Can you work these out from the model? Positions are in its coordinate system, mm. A direction names the side the tool comes from. Coordinates: 2 decimals unless noted, no trailing zeros. Loops run counter-clockwise (first coordinate to the right, second up) from the corner with the lowest first, then second, coordinate; pieces in that order, holes last. Notation, with made-up numbers: M 65.5,36 L 96.5,36 A26 ccw 96.5,53 Z; hole C -19.75,32 d5. An arc over 180 degrees is marked long. Answer as a JSON object with one key per item and string values. Group by question number.
Item 1: If I drill on line 1 (Z direction, x = 25.4, y = 3.25); line 2 (X direction, y = 8.5, z = -73); line 3 (X direction, y = 7, z = -31.75), over which ranges is the centre line in solid material (lowest first)?
Item 2: Which directions (+Z, -Z, +X, -X, +Y, -Y) give clear straight access to the entire face, cutting with the end or side of a thin tool? Please do faces 3 (the flat face through (684, 0, -177)), 4 (the flat face through (295.988, 5.009, -186.063)).
Item 3: We'd pull the mould along X, two halves only. Please class faces 1 (the flat face through (1165.75, 5.01, -178.62)), 2 (the flat face through (684, 10.16, -177)): +X half, -X half, draft (parallel to the pull), parting line (faces both ways), or undercut.
Item 4: I'm going to push a flat-ended pin straight in: pin 1 Ø7.5 at (x, z) = (1361.53, -31.75) entering from +Y. Where does the tip first touch, or does it pass through?
Item 5: Suppose I cut it at A-A (x = 337.5). Write out the boundary of the cut face in (y, z).
Item 6: Suppose I cut it at B-B (y = 2.25). Count the separate pieces of the cut face and the enclosed holes in it, then the cut area to 3 significant figures.
```python
from build123d import *

# Parameters (mm, degrees)
SKETCH1_W           = 1386.9289
SKETCH1_H           = 349.25
SKETCH1_W_2         = 1285.3289
SKETCH1_H_2         = 247.65
BOSS_EXTRUDE1_DEPTH = 10.16
FILLET1_R           = 19.05
SKETCH4_R           = 4.7625
CUT_EXTRUDE1_DEPTH  = 11.16


with BuildPart() as part:
    # Sketch1 → Boss-Extrude1 (new body)
    with BuildSketch(Plane(origin=(0, 0, 0), x_dir=(1, 0, 0), z_dir=(0, 1, 0))):
        with Locations((693.46445, 174.625)):
            Rectangle(SKETCH1_W, SKETCH1_H)
        with Locations((693.46445, 174.625)):
            Rectangle(SKETCH1_W_2, SKETCH1_H_2, mode=Mode.SUBTRACT)
        Polygon((453.842966667, 65.481790785), (50.8, 298.45), (50.8, 269.112055616), (428.487319876, 50.8), (453.842966667, 50.8), align=None)
        Polygon((101.55564679, 298.45), (50.8, 298.45), (453.842966667, 65.481790785), (453.842966667, 94.819735169), align=None)
        Polygon((453.842966667, 94.819735169), (453.842966667, 65.481790785), (453.842966667, 50.8), (479.242966667, 50.8), (479.242966667, 298.45), (453.842966667, 298.45), align=None)
        Polygon((504.642966667, 298.45), (479.242966667, 298.45), (479.242966667, 50.8), (504.642966667, 50.8), (504.642966667, 65.481790785), (504.642966667, 94.819735169), align=None)
        Polygon((882.285933333, 298.45), (856.930286543, 298.45), (504.642966667, 94.819735169), (504.642966667, 65.481790785), (882.285933333, 283.768209215), align=None)
        Polygon((504.642966667, 65.481790785), (504.642966667, 50.8), (529.998613457, 50.8), (882.285933333, 254.430264831), (882.285933333, 283.768209215), align=None)
        Polygon((907.685933333, 298.45), (882.285933333, 298.45), (882.285933333, 283.768209215), (882.285933333, 254.430264831), (882.285933333, 50.8), (907.685933333, 50.8), align=None)
        Polygon((933.085933333, 298.45), (907.685933333, 298.45), (907.685933333, 50.8), (933.085933333, 50.8), (933.085933333, 254.430264831), (933.085933333, 283.768209215), align=None)
        Polygon((1336.1289, 50.8), (933.085933333, 283.768209215), (933.085933333, 254.430264831), (1285.37325321, 50.8), align=None)
        Polygon((958.441580124, 298.45), (933.085933333, 298.45), (933.085933333, 283.768209215), (1336.1289, 50.8), (1336.1289, 80.137944384), align=None)
    extrude(amount=BOSS_EXTRUDE1_DEPTH)

    # Fillet1
    fillet1_edges = [part.edges().sort_by_distance(p)[0] for p in [
        (428.487319876, 5.08, -50.8),
        (50.8, 5.08, -269.112055616),
        (50.8, 5.08, -50.8),
        (1336.1289, 5.08, -80.137944384),
        (1336.1289, 5.08, -298.45),
        (958.441580124, 5.08, -298.45),
        (856.930286543, 5.08, -298.45),
        (504.642966667, 5.08, -298.45),
        (504.642966667, 5.08, -94.819735169),
        (453.842966667, 5.08, -298.45),
        (101.55564679, 5.08, -298.45),
        (453.842966667, 5.08, -94.819735169),
        (529.998613457, 5.08, -50.8),
        (882.285933333, 5.08, -50.8),
        (882.285933333, 5.08, -254.430264831),
        (933.085933333, 5.08, -50.8),
        (1285.37325321, 5.08, -50.8),
        (933.085933333, 5.08, -254.430264831),
    ]]
    fillet(fillet1_edges, radius=FILLET1_R)

    # Sketch4 → Cut-Extrude1 (cut, through all)
    with BuildSketch(Plane(origin=(0, 10.16, 0), x_dir=(1, 0, 0), z_dir=(0, 1, 0))):
        with Locations((25.4, 317.5)):
            Circle(SKETCH4_R)
        with Locations((25.4, 238.125)):
            Circle(SKETCH4_R)
        with Locations((25.4, 111.125)):
            Circle(SKETCH4_R)
        with Locations((25.4, 31.75)):
            Circle(SKETCH4_R)
        with Locations((1361.5289, 31.75)):
            Circle(SKETCH4_R)
        with Locations((1361.5289, 111.125)):
            Circle(SKETCH4_R)
        with Locations((1361.5289, 238.125)):
            Circle(SKETCH4_R)
        with Locations((1361.5289, 317.5)):
            Circle(SKETCH4_R)
    extrude(amount=-CUT_EXTRUDE1_DEPTH, mode=Mode.SUBTRACT)


solid = part.part
```
From the geometry:
{
 "1": {"line 1": "-349.25 to -322.26, -312.74 to -242.89, -233.36 to -115.89, -106.36 to -36.51, -26.99 to 0", "line 2": "0 to 50.8, 376.25 to 582.23, 882.29 to 933.09, 1233.14 to 1386.93", "line 3": "0 to 20.64, 30.16 to 1356.77, 1366.29 to 1386.93"},
 "2": {"face 3": "+Z, -Z, +X, -X, -Y", "face 4": "+Y, -Y"},
 "3": {"face 1": "undercut", "face 2": "draft"},
 "4": {"pin 1": "through"},
 "5": {"outline": "M 0,-349.25 L 10.16,-349.25 L 10.16,-298.45 L 0,-298.45 Z; M 0,-162.07 L 10.16,-162.07 L 10.16,-103.39 L 0,-103.39 Z; M 0,-50.8 L 10.16,-50.8 L 10.16,0 L 0,0 Z"},
 "6": {"separate pieces": "1", "enclosed holes": "14", "area": "265,000 mm2"}
}
